```python
from build123d import *

# Parameters (mm, degrees)
F1_DEPTH = 300
F2_R     = 10


with BuildPart() as f1:
    # F0 (on Front) → F1 (new body, symmetric)
    with BuildSketch(Plane.XZ):
        with BuildLine():
            Line((-201.5, 1.5), (-201.5, 0))
            Line((-201.5, 0), (-3.5, 0))
            ThreePointArc((-3.5, 0), (-1.025126, 1.025126), (0, 3.5))
            Line((0, 3.5), (0, 101.5))
            Line((0, 101.5), (-1.5, 101.5))
            Line((-1.5, 101.5), (-1.5, 3.5))
            ThreePointArc((-1.5, 3.5), (-2.085786, 2.085786), (-3.5, 1.5))
            Line((-3.5, 1.5), (-201.5, 1.5))
        make_face()
    extrude(amount=F1_DEPTH, both=True)

    # F2
    f2_edges = [f1.edges().sort_by_distance(p)[0] for p in [
        (-0.75, -300, 101.5),
        (-0.75, 300, 101.5),
        (-201.5, -300, 0.75),
        (-201.5, 300, 0.75),
    ]]
    fillet(f2_edges, radius=F2_R)


solid = f1.part
```
Build history of the part. All positions in model axes, mm. A direction names the side the tool comes from. Give positions to 0.01 mm unless a question says otherwise; leave off trailing zeros. Order: outer loops, then holes, each group sorted by start corner. A loop starts at its lowest first (then second) coordinate and runs counter-clockwise, first axis right, second up. Notation, with made-up numbers: M 31,-9 L 53,-9 A29 ccw 53,28 Z; hole C -13,82 d2. An arc over 180 degrees is marked long. Write item = value, one per line. Start each with the question number.
(1) Slice it at A-A on y = -172. Write the cut outline in (x, z), plus the area to 3 significant figures.
(2) Pin check, flat tips, straight feed: pin 1 Ø1 at (y, z) = (163, 25.5) entering from -X; pin 2 Ø5 at (x, y) = (-110, 57) entering from +Z. Stop position of each tip, or through.
(3) Which spindle directions (+Z, -Z, +X, -X, +Y, -Y) get a long thin tool onto all of the face, cutting with end or side? Do faces 1 (the flat face through (0, -4, 52)), 2 (the flat face through (-101, -4, 1.5)). Say none if no direction does.
(4) Probe L1, parallel to X at y = 102, z = 66; L2, parallel to Z at x = -18, y = 50. List the from-to ranges inside material, lowest first. Write a range as [from, to].
(5) Slice it at B-B on x = -84.5. Write the cut outline in (y, z).
(6) Slice it at C-C on z = 43.5. Write the cut outline in (x, y), plus the area to 3 significant figures.
Responses:
q1.outline = M -201.5,0 L -3.5,0 A3.5 ccw 0,3.5 L 0,101.5 L -1.5,101.5 L -1.5,3.5 A2 cw -3.5,1.5 L -201.5,1.5 Z
q1.area = 450 mm2
q2.pin_1 = -1.5
q2.pin_2 = 1.5
q3.face_1 = +Z, -Z, +X, +Y, -Y
q3.face_2 = +Z, -X, +Y, -Y
q4.L1 = [-1.5, 0]
q4.L2 = [0, 1.5]
q5.outline = M -300,0 L 300,0 L 300,1.5 L -300,1.5 Z
q6.outline = M -1.5,-300 L 0,-300 L 0,300 L -1.5,300 Z
q6.area = 900 mm2
